```python
from build123d import *

# Parameters (mm, degrees)
F1_DEPTH = 32


with BuildPart() as f1:
    # F0 (on Front) → F1 (new body)
    with BuildSketch(Plane.XZ):
        with BuildLine():
            ThreePointArc((61.773781, 67.5), (91.5, 0), (61.773781, -67.5))
            Line((61.773781, -67.5), (66.616439, -67.5))
            ThreePointArc((66.616439, -67.5), (70.779316, -66.592329), (74.186489, -64.034091))
            ThreePointArc((74.186489, -64.034091), (98, 0), (74.186489, 64.034091))
            ThreePointArc((74.186489, 64.034091), (70.779316, 66.592329), (66.616439, 67.5))
            Line((66.616439, 67.5), (61.773781, 67.5))
        make_face()
    extrude(amount=F1_DEPTH)


solid = f1.part
```
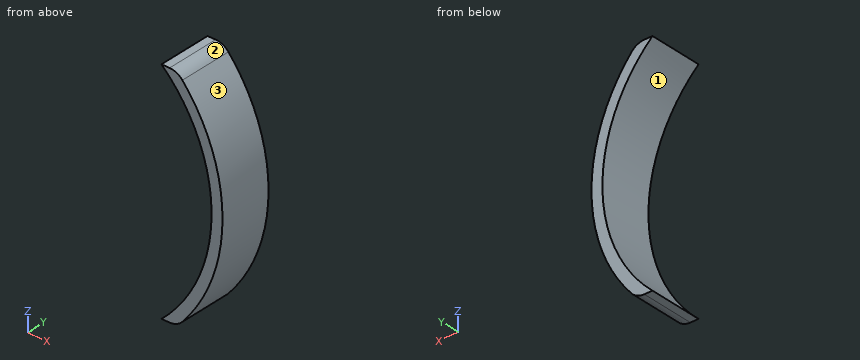
Design review of the part built by this model. Coordinates are the model's own, in mm. Face numbers are marked on the shaded views. Round coordinates to 2 decimals unless told otherwise and drop trailing zeros. Write each loop counter-clockwise with the first axis right and the second up, starting at its lowest first coordinate (ties: lowest second). Pieces come first, ordered by that corner, then holes.
Item 1: For probe 1 along Z at (x, y) = (78.5, -4); probe 2 along Z at (x, y) = (80, -30); probe 3 along X at (y, z) = (-14.5, 35), list the stretches that pass through material, from the lowest coordinate up.
Item 2: We need section A-A on x = 79.5. Write out the cut boundary in (y, z), and give its area (3 significant figures).
Item 3: We need section B-B on y = -23. Write out the cut boundary in (x, z).
Item 4: The part is to be moulded in two halves that separate along Z. For the marked faces 1, 2 and 3, say which applies: +Z half, -Z half, draft (parallel to the pull), parting line (faces both ways), or undercut.
Item 5: We need section D-D on z = 6. Write out the cut boundary in (x, y), and give its area (3 significant figures).
Item 6: Clearance check with flat-ended pins moving along their axes: pin 1 Ø6 at (x, y) = (92, -10) entering from -Z; pin 2 Ø12 at (x, y) = (89, -22.5) entering from -Z; pin 3 Ø1 at (y, z) = (-8.5, 35.5) entering from -X. State where each tip first meets the part, or that it passes through.
Item 7: We need section C-C on x = 88.5. Write out the cut boundary in (y, z), and give its area (3 significant figures).
Returned:
1. probe 1: z = -58.67 to -47.01, 47.01 to 58.67
1. probe 2: z = -56.6 to -44.41, 44.41 to 56.6
1. probe 3: x = 84.54 to 91.54
2. outline: (-32, -57.3) - (0, -57.3) - (0, -45.3) - (-32, -45.3) - close; (-32, 45.3) - (0, 45.3) - (0, 57.3) - (-32, 57.3) - close
2. area: 768 mm2
3. outline: (61.77, -67.5) - (66.62, -67.5) arc R10 ccw to (74.19, -64.03) arc R98 ccw to (74.19, 64.03) arc R10 ccw to (66.62, 67.5) - (61.77, 67.5) arc R91.5 cw to start
4. face 1: undercut
4. face 2: +Z half
4. face 3: parting line
5. outline: (91.3, -32) - (97.82, -32) - (97.82, 0) - (91.3, 0) - close
5. area: 208 mm2
6. pin 1: stops at z = -41.02
6. pin 2: stops at z = -52.11
6. pin 3: stops at x = 84.12
7. outline: (-32, -42.09) - (0, -42.09) - (0, -23.24) - (-32, -23.24) - close; (-32, 23.24) - (0, 23.24) - (0, 42.09) - (-32, 42.09) - close
7. area: 1,210 mm2
